from build123d import *

# Parameters (mm, degrees)
F1_DEPTH = 430
F2_ANGLE = 25


with BuildPart() as f1:
    # F0 (on Front) → F1 (new body)
    with BuildSketch(Plane.XZ):
        with BuildLine():
            Line((-43.73349, 41.551889), (-43.73349, 38.551889))
            Line((-43.73349, 38.551889), (28.26651, 38.551889))
            ThreePointArc((28.26651, 38.551889), (30.38783, 37.673209), (31.26651, 35.551889))
            Line((31.26651, 35.551889), (31.26651, -50.448111))
            ThreePointArc((31.26651, -50.448111), (30.38783, -52.569431), (28.26651, -53.448111))
            Line((28.26651, -53.448111), (-43.73349, -53.448111))
            Line((-43.73349, -53.448111), (-43.73349, -56.448111))
            Line((-43.73349, -56.448111), (28.26651, -56.448111))
            ThreePointArc((28.26651, -56.448111), (32.509151, -54.690752), (34.26651, -50.448111))
            Line((34.26651, -50.448111), (34.26651, 35.551889))
            ThreePointArc((34.26651, 35.551889), (32.509151, 39.79453), (28.26651, 41.551889))
            Line((28.26651, 41.551889), (-43.73349, 41.551889))
        make_face()
    extrude(amount=-F1_DEPTH)


with BuildPart() as f1_1:
    # F2: moved
    add(f1.part.rotate(Axis((-43.73349, 0, 40.051889), (0, 0, -1)), F2_ANGLE))


solid = f1_1.part
Design review of the part built by this model. Coordinates are the model's own, in mm. A direction names the side the tool comes from. Coordinates: 2 decimals unless noted, no trailing zeros. Loops run counter-clockwise (first coordinate to the right, second up) from the corner with the lowest first, then second, coordinate; pieces in that order, holes last.
Item 1: For faces 5 (the flat face through (45.86, 192.13, 40.07)), 6 (the flat face through (113.83, 160.43, -6.85)), list the 3-axis set-ups (+Z, -Z, +X, -X, +Y, -Y) from which the entire face can be reached by the end or side of a thin tool; tool diameter is ignored.
Completed:
face 5: +Z, -Z, -X, +Y
face 6: -X, +Y
Item 2: Add section A-A (x = -13). Write out the cut boundary in (y, z).
Completed:
outline: (-14.33, -56.45) - (65.91, -56.45) - (65.91, -53.45) - (-14.33, -53.45) - close; (-14.33, 38.55) - (65.91, 38.55) - (65.91, 41.55) - (-14.33, 41.55) - close
Item 3: Add section B-B (z = -8). Write out the cut boundary in (x, y).
Completed:
outline: (24.24, -31.7) - (26.96, -32.96) - (208.68, 356.75) - (205.97, 358.02) - close
Item 4: Add section C-C (x = 14.5). Write out the cut boundary in (y, z).
Completed:
outline: (-27.15, -56.45) - (124.88, -56.45) - (124.88, -53.45) - (-27.15, -53.45) - close; (-27.15, 38.55) - (124.88, 38.55) - (124.88, 41.55) - (-27.15, 41.55) - close
Item 5: Draft analysis for pull direction Z (two halves, no side actions). For faces 1 (the flat face through (79, 177, -53.448)), 2 (the cylindrical face through (115, 159.89, 39.75)), 3 (the flat face through (78, 177, 38.552)), 4 (the flat face through (116.549, 159.164, -8.05)), state which applies: pulls with the +Z half, pulls with the -Z half, needs draft (parallel to the pull), parting line crosses it, or undercut.
Completed:
face 1: undercut
face 2: pulls with the +Z half
face 3: undercut
face 4: needs draft
Item 6: Clearance check with flat-ended pins moving along their axes: pin 1 (1 mm diameter, centred on y = 269.5, z = -39.5, fed in from +X); pin 2 (10 mm diameter, centred on x = 173, z = -33, fed in from +Y). State where each tip first meets the part, or that it passes through.
Completed:
pin 1: stops at x = 168.23
pin 2: stops at y = 298.04
Item 7: Wall thickness on L1, parallel to Z at x = 81.5, y = 156; L2, parallel to Y at x = 183, z = -16.5; L3, parallel to Y at x = 140, z = 3: over which ranges is each line inside the solid? List them lowest first.
Completed:
L1: z = -56.45 to -53.45, 38.55 to 41.55
L2: y = 301.67 to 308.77
L3: y = 209.45 to 216.55
